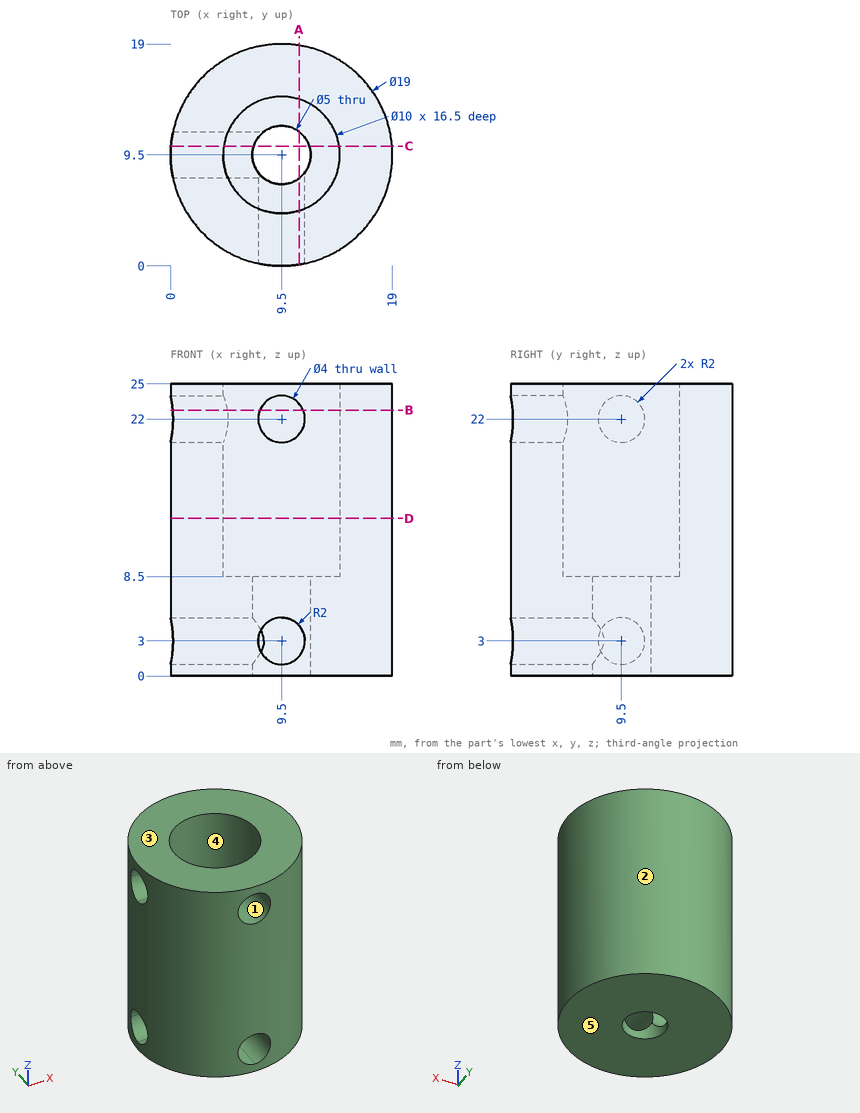
Design review of the part shown in the three views and the two pictorial views. Dimensions are in mm from the part's minimum x, y and z. A direction names the side the tool comes from. Round coordinates to 2 decimals unless told otherwise and drop trailing zeros. Write each loop counter-clockwise with the first axis right and the second up, starting at its lowest first coordinate (ties: lowest second). Pieces come first, ordered by that corner, then holes. Notation, with made-up numbers: (73, 77.5) - (113, 77.5) arc R15 cw to (113, 100.5) - close; hole circle Ø10 at (14, 89). An arc over 180 degrees is marked (long way). Return JSON: item names as keys, results as strings. Group by question number.
Item 1: We need section D-D on z = 13.5. Write out the cut boundary in (x, y), and give its area (3 significant figures).
Item 2: We need section C-C on y = 10.25. Write out the cut boundary in (x, z), and give its area (3 significant figures).
Item 3: We need section B-B on z = 22.75. Write out the cut boundary in (x, y), and give its area (3 significant figures).
Item 4: We need section A-A on x = 11. Write out the cut boundary in (y, z), and give its area (3 significant figures).
Item 5: For probe 1 along Z at (x, y) = (10, 4); probe 2 along X at (y, z) = (11.75, 12.5); probe 3 along Z at (x, y) = (12.25, 7), list the stretches that pass through material, from the lowest coordinate up. Write a range as [from, to].
Item 6: Machinability: for the marked faces 4 and 5, which of the approach directions +Z, -Z, +X, -X, +Y, -Y give a long, thin tool a straight path to every point of the face, cutting with its end or side? Answer none if there is none.
Item 7: The part is to be moulded in two halves that separate along X. For the marked faces 1, 2 and 3, say which applies: pulls with the +X half, pulls with the -X half, needs draft (parallel to the pull), parting line crosses it, or undercut.
Item 8: Insertion check: P1, Ø8, axis at x = 9.5, y = 9.5, coming from the +Z side; P2, Ø6, axis at y = 13, z = 19.5, coming from the -X side; P3, Ø2, axis at y = 14.5, z = 16.5, coming from the -X side. Each pin has a flat end and moves straight along its axis. Give the tip position at first contact, or say it passes through.
Model answer:
{
 "1": {"outline": "circle Ø19 at (9.5, 9.5); hole circle Ø10 at (9.5, 9.5)", "area": "205 mm²"},
 "2": {"outline": "(0.03, 0) - (7.12, 0) - (7.12, 1.15) - (0.03, 1.15) - close; (0.03, 4.85) - (7.12, 4.85) - (7.12, 8.5) - (4.56, 8.5) - (4.56, 20.15) - (0.03, 20.15) - close; (0.03, 23.85) - (4.56, 23.85) - (4.56, 25) - (0.03, 25) - close; (11.88, 0) - (18.97, 0) - (18.97, 25) - (14.44, 25) - (14.44, 8.5) - (11.88, 8.5) - close", "area": "227 mm²"},
 "3": {"outline": "(0.18, 7.65) arc R9.5 ccw to (7.65, 0.18) - (7.65, 4.86) arc R5 cw to (4.86, 7.65) - close; (0.18, 11.35) - (4.86, 11.35) arc R5 cw (long way) to (11.35, 4.86) - (11.35, 0.18) arc R9.5 ccw (long way) to start", "area": "171 mm²"},
 "4": {"outline": "(0.12, 0) - (7.5, 0) - (7.5, 1.68) - (0.12, 1.68) - close; (0.12, 4.32) - (7.5, 4.32) - (7.5, 8.5) - (4.73, 8.5) - (4.73, 20.68) - (0.12, 20.68) - close; (0.12, 23.32) - (4.73, 23.32) - (4.73, 25) - (0.12, 25) - close; (11.5, 0) - (18.88, 0) - (18.88, 25) - (14.27, 25) - (14.27, 8.5) - (11.5, 8.5) - close", "area": "246 mm²"},
 "5": {"probe 1": "z = [0, 1.06], [4.94, 20.06], [23.94, 25]", "probe 2": "x = [0.27, 5.03], [13.97, 18.73]", "probe 3": "z = [0, 8.5]"},
 "6": {"face 4": "+Z", "face 5": "-Z, +X, -X, +Y, -Y"},
 "7": {"face 1": "undercut", "face 2": "parting line crosses it", "face 3": "needs draft"},
 "8": {"P1": "stops at z = 8.5", "P2": "stops at x = 0.01", "P3": "stops at x = 0.88"}
}
